Work out the finished part from the listing and answer in its coordinate system (mm). Face numbers are marked on the shaded views. A direction names the side the tool comes from. Round coordinates to 2 decimals unless told otherwise and drop trailing zeros. Order: outer loops, then holes, each group sorted by start corner. A loop starts at its lowest first (then second) coordinate and runs counter-clockwise, first axis right, second up. Notation, with made-up numbers: M 17.5,70 L 48.5,70 A30 ccw 48.5,101 Z; hole C 45,-17.75 d7. An arc over 180 degrees is marked long. Return JSON: item names as keys, results as strings.
from build123d import *

# Parameters (mm, degrees)
SKETCH2_R                                       = 6.35
BOSS_EXTRUDE3_DEPTH                             = 3.175
BOSS_EXTRUDE4_DEPTH                             = 3.175
BOSS_EXTRUDE5_DEPTH                             = 1.019725
CSK_FOR_4_FLAT_HEAD_MACHINE_SCREW_4_D           = 3.2639
CSK_FOR_4_FLAT_HEAD_MACHINE_SCREW_4_DEPTH       = 3.175
CSK_FOR_4_FLAT_HEAD_MACHINE_SCREW_4_CSINK_D     = 5.715
CSK_FOR_4_FLAT_HEAD_MACHINE_SCREW_4_CSINK_ANGLE = 100


# Read off the part's stored shape, not the designer's step: CSK for #4 Flat Head Machine Screw (100)1
with BuildPart() as part:
    # Sweep1: sweep along a path in Sketch5
    with BuildLine(Plane(origin=(0, 0, 0), x_dir=(0, 0, -1), z_dir=(1, 0, 0))) as sweep1_path:
        Line((0, 0), (0, 40))
        Line((0, 40), (40, 40))
    # Sketch2 → Sweep1 (sweep)
    with BuildSketch(Plane(origin=(0, 0, 0), x_dir=(1, 0, 0), z_dir=(0, 1, 0))):
        with BuildLine():
            Line((-3.684990204, -8.783413773), (3.684734386, -8.783413773))
            ThreePointArc((3.684734386, -8.783413773), (9.525, 0), (3.684734386, 8.783413773))
            Line((3.684734386, 8.783413773), (-3.684990204, 8.783413773))
            ThreePointArc((-3.684990204, 8.783413773), (-9.525098966, 0), (-3.684990204, -8.783413773))
        make_face()
        Circle(SKETCH2_R, mode=Mode.SUBTRACT)
    sweep(path=sweep1_path.line, transition=Transition.RIGHT)

    # CSK for _4 Flat Head Machine Screw _ 2 → CSK for _4 Flat Head Machine Screw _100 (revolve, cut)
    with BuildSketch(Plane(origin=(-0.000127909, 0, -15.608293114), x_dir=(1, 0, 0), z_dir=(0, 0, 1))):
        Polygon((0, 46.136589997), (1.63195, 46.136589997), (1.63195, 47.75505522), (2.8575, 48.783413773), (0, 48.783413773), align=None)
    revolve(axis=Axis((-0.000127909, 0, -15.608293114), (0, 1, 0)), mode=Mode.SUBTRACT)

    # CSK for _4 Flat Head Machine Screw _ 3 o → CSK for _4 Flat Head Machine Screw _ 3 (revolve, cut)
    with BuildSketch(Plane(origin=(-6.3954e-05, 24.391706886, 0), x_dir=(1, 0, 0), z_dir=(0, -1, 0))):
        Polygon((0, 6.13660701), (1.63195, 6.13660701), (1.63195, 7.75505522), (2.8575, 8.783413773), (0, 8.783413773), align=None)
    revolve(axis=Axis((-6.3954e-05, 24.391706886, 0), (0, 0, 1)), mode=Mode.SUBTRACT)

    # Sketch13 → Boss-Extrude3 (add)
    with BuildSketch(Plane(origin=(-3.684990204, 0, 0), x_dir=(0, 0, -1), z_dir=(1, 0, 0))):
        with BuildLine():
            ThreePointArc((11.983413773, 0.164448528), (30.85687358, 9.14312642), (39.835551472, 28.016586227))
            Line((39.835551472, 28.016586227), (11.983413773, 28.016586227))
            Line((11.983413773, 28.016586227), (11.983413773, 0.164448528))
        make_face()
        with BuildLine():
            Line((40, 31.216586227), (8.783413773, 31.216586227))
            Line((8.783413773, 31.216586227), (8.783413773, 0))
            ThreePointArc((8.783413773, 0), (10.385525139, 0.04113924), (11.983413773, 0.164448528))
            Line((11.983413773, 0.164448528), (11.983413773, 28.016586227))
            Line((11.983413773, 28.016586227), (39.835551472, 28.016586227))
            ThreePointArc((39.835551472, 28.016586227), (39.95886076, 29.614474861), (40, 31.216586227))
        make_face()
    extrude(amount=BOSS_EXTRUDE3_DEPTH)

    # Sketch15 → Boss-Extrude4 (add)
    with BuildSketch(Plane(origin=(-0.509990204, 0, 0), x_dir=(0, 0, -1), z_dir=(1, 0, 0))):
        with BuildLine():
            Line((8.783413773, 31.216586227), (40, 31.216586227))
            ThreePointArc((40, 31.216586227), (39.95886076, 29.614474861), (39.835551472, 28.016586227))
            Line((39.835551472, 28.016586227), (11.983413773, 28.016586227))
            Line((11.983413773, 28.016586227), (11.983413773, 0.164448528))
            ThreePointArc((11.983413773, 0.164448528), (10.385525139, 0.04113924), (8.783413773, 0))
            Line((8.783413773, 0), (8.783413773, 31.216586227))
        make_face()
    extrude(amount=BOSS_EXTRUDE4_DEPTH)

    # Sketch16 → Boss-Extrude5 (add)
    with BuildSketch(Plane(origin=(2.665009796, 0, 0), x_dir=(0, 0, -1), z_dir=(1, 0, 0))):
        with BuildLine():
            Line((8.783413773, 31.216586227), (40, 31.216586227))
            ThreePointArc((40, 31.216586227), (30.85687358, 9.14312642), (8.783413773, 0))
            Line((8.783413773, 0), (8.783413773, 31.216586227))
        make_face()
    extrude(amount=BOSS_EXTRUDE5_DEPTH)

    # CSK for _4 Flat Head Machine Screw _ 4
    with Locations(Plane.ZY.offset(3.684990204)):
        with Locations((-27.511452395, 21.903897361), (-18.096102639, 12.488547605)):
            CounterSinkHole(CSK_FOR_4_FLAT_HEAD_MACHINE_SCREW_4_D / 2, CSK_FOR_4_FLAT_HEAD_MACHINE_SCREW_4_CSINK_D / 2, depth=CSK_FOR_4_FLAT_HEAD_MACHINE_SCREW_4_DEPTH, counter_sink_angle=CSK_FOR_4_FLAT_HEAD_MACHINE_SCREW_4_CSINK_ANGLE)


solid = part.part
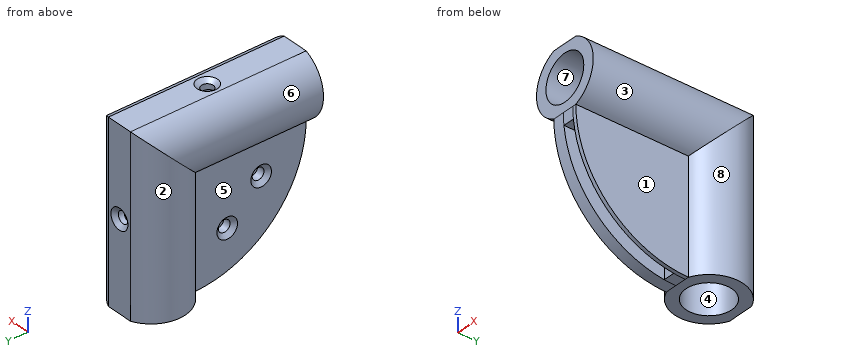
Item 1: Find section C-C (y = 40). Determine the outline of the cut face in (x, z) (3 decimals).
Output:
{"outline": "M -9.525,-40 L -6.35,-40 L -6.35,0 A6.35 cw 6.35,0 L 6.35,-40 L 9.525,-40 L 9.525,0 A9.525 ccw 3.685,8.783 L -3.685,8.783 A9.525 ccw -9.525,0 Z"}
Item 2: Find section A-A (z = -37). Determine the outline of the cut face in (x, y) (3 decimals), plus the area to 3 significant figures.
Output:
{"outline": "M -3.685,17.864 L -0.51,17.864 L -0.51,28.017 L 2.665,28.017 L 2.665,17.864 L 3.685,17.864 L 3.685,31.217 A9.525 ccw 3.685,48.783 L -3.685,48.783 A9.525 ccw -3.685,31.217 Z; hole C 0,40 d12.7", "area": "217 mm^2"}
Item 3: Find section D-D (z = 0). Determine the outline of the cut face in (x, y) (3 decimals), plus the area to 3 significant figures.
Output:
{"outline": "M -9.525,0 L -6.35,0 L -6.35,40 A6.35 cw 6.35,40 L 6.35,0 L 9.525,0 L 9.525,40 A9.525 ccw 3.685,48.783 L -3.685,48.783 A9.525 ccw -9.525,40 Z", "area": "330 mm^2"}
Item 4: Each of these flat-tipped pins is pushed along its axis until it touches: pin 1 (6 mm diameter, centred on y = 18.5, z = -28, fed in from -X) (3 decimals); pin 2 (25 mm diameter, centred on y = 17.5, z = -32, fed in from +X); pin 3 (1.5 mm diameter, centred on x = -4.5, y = 13, fed in from +Z); pin 4 (3 mm diameter, centred on y = 34.5, z = 1.5, fed in from +X) (3 decimals). Where does it stop, or does it pass through?
Output:
{"pin 1": "stops at x = -3.685", "pin 2": "stops at x = 3.68", "pin 3": "stops at z = 8.76", "pin 4": "stops at x = 9.525"}
Item 5: Find section B-B (y = 18). Determine the outline of the cut face in (x, z) (3 decimals).
Output:
{"outline": "M -3.685,-37.064 L -0.51,-37.064 L -0.51,-11.983 L 2.665,-11.983 L 2.665,-37.064 L 3.685,-37.064 L 3.685,-8.783 A9.525 ccw 3.685,8.783 L -3.685,8.783 A9.525 ccw -3.685,-8.783 Z; hole C 0,0 d12.7"}
Item 6: The mould has two halves that part along X. Classify the marked faces 6, 7 and 8: pulls with the +X half, pulls with the -X half, needs draft (parallel to the pull), parting line crosses it, or undercut.
Output:
{"face 6": "pulls with the -X half", "face 7": "undercut", "face 8": "pulls with the +X half"}
Item 7: Which of the six approach directions +Z, -Z, +X, -X, +Y, -Y give full straight-line access (tool end or side, diameter ignored) to the marked faces 1, 2, 3, 4 and 5?
Output:
{"face 1": "-Z, +X, -Y", "face 2": "-Z, -X", "face 3": "+X, -Y", "face 4": "-Z", "face 5": "-Z, -X, -Y"}
Item 8: Consider line 1 along Z through (x, y) = (0, 27.5); line 2 along Y through (x, z) = (-2, -27); line 3 along X through (y, z) = (18.5, -21) (3 decimals). Determine where each line is inside the solid, lowest interval first. Write a range as [from, to].
Output:
{"line 1": "z = [-11.98, -6.35], [6.35, 8.78]", "line 2": "y = [5.87, 20.35], [23.45, 33.97], [46.03, 48.78]", "line 3": "x = [-3.685, -0.51], [2.665, 3.685]"}
